Part model, mm, in its own coordinate system. A direction names the side the tool comes from. Round coordinates to 2 decimals unless told otherwise and drop trailing zeros. Write each loop counter-clockwise with the first axis right and the second up, starting at its lowest first coordinate (ties: lowest second). Pieces come first, ordered by that corner, then holes.
```python
from build123d import *

# Parameters (mm, degrees)
F1_DEPTH = 13
F3_DEPTH = 25
F5_DEPTH = 25


with BuildPart() as f1:
    # F0 (on Front) → F1 (new body)
    with BuildSketch(Plane.XZ):
        with BuildLine():
            Line((109.81556, 142.312214), (-107.18444, 142.312214))
            ThreePointArc((-107.18444, 142.312214), (-135.468711, 130.596485), (-147.18444, 102.312214))
            Line((-147.18444, 102.312214), (-147.18444, -27.687786))
            ThreePointArc((-147.18444, -27.687786), (-135.468711, -55.972058), (-107.18444, -67.687786))
            Line((-107.18444, -67.687786), (109.81556, -67.687786))
            ThreePointArc((109.81556, -67.687786), (138.099831, -55.972058), (149.81556, -27.687786))
            Line((149.81556, -27.687786), (149.81556, 102.312214))
            ThreePointArc((149.81556, 102.312214), (138.099831, 130.596485), (109.81556, 142.312214))
        make_face()
    extrude(amount=F1_DEPTH)

    # F2 (on face) → F3 (cut)
    with BuildSketch(Plane.XZ.offset(13)):
        with BuildLine():
            Line((149.81556, -27.687786), (149.81556, -4.202998))
            Line((149.81556, -4.202998), (0, -4.202998))
            Line((0, -4.202998), (0, -30.806687))
            Line((0, -30.806687), (149.693781, -30.806687))
            ThreePointArc((149.693781, -30.806687), (149.785104, -29.248425), (149.81556, -27.687786))
        make_face()
    extrude(amount=-F3_DEPTH, mode=Mode.SUBTRACT)

    # F4 (on face) → F5 (cut)
    with BuildSketch(Plane.XZ.offset(13)):
        with BuildLine():
            Line((36.957689, 109.959573), (149.077729, 109.959573))
            ThreePointArc((149.077729, 109.959573), (147.134331, 116.710454), (144.039855, 123.017229))
            Line((144.039855, 123.017229), (36.957689, 123.017229))
            Line((36.957689, 123.017229), (36.957689, 109.959573))
        make_face()
    extrude(amount=-F5_DEPTH, mode=Mode.SUBTRACT)


solid = f1.part
```
Q1. Mould opens along Z. For faces 3 (the cylindrical face through (-135.156, -6.409, 130.906)), 4 (the flat face through (0, -7, -17)), 5 (the flat face through (149.816, -6, 48)) say: +Z half, -Z half, draft (parallel to the pull), parting line (faces both ways), or undercut.
Values follow:
face 3: +Z half
face 4: undercut
face 5: draft
Q2. Wall check: L1, parallel to Z at x = 64, y = -6.25; L2, parallel to Z at x = 7, y = -2.5; L3, parallel to Z at x = 133, y = -4.5. Give the ranges that are in metal, low to high.
Values follow:
L1: z = -67.69 to -30.81, -4.2 to 109.96, 123.02 to 142.31
L2: z = -67.69 to -30.81, -4.2 to 142.31
L3: z = -60.28 to -30.81, -4.2 to 109.96, 123.02 to 134.91
Q3. Cut at C-C on y = -6. Write the cut outline in (x, z), plus the area to 3 significant figures.
Values follow:
outline: (-147.18, -27.69) arc R40 ccw to (-107.18, -67.69) - (109.82, -67.69) arc R40 ccw to (149.69, -30.81) - (0, -30.81) - (0, -4.2) - (149.82, -4.2) - (149.82, 102.31) arc R40 ccw to (149.08, 109.96) - (36.96, 109.96) - (36.96, 123.02) - (144.04, 123.02) arc R40 ccw to (109.82, 142.31) - (-107.18, 142.31) arc R40 ccw to (-147.18, 102.31) - close
area: 55,600 mm2
Q4. Cut at A-A on x = 100. Write the cut outline in (y, z).
Values follow:
outline: (-13, -67.69) - (0, -67.69) - (0, -30.81) - (-13, -30.81) - close; (-13, -4.2) - (0, -4.2) - (0, 109.96) - (-13, 109.96) - close; (-13, 123.02) - (0, 123.02) - (0, 142.31) - (-13, 142.31) - close
Q5. Which spindle directions (+Z, -Z, +X, -X, +Y, -Y) get a long thin tool onto all of the face, cutting with end or side? Do faces 1 (the flat face through (-147.184, -6, 38)), 2 (the flat face through (91, -7, 123.017)). Say none if no direction does.
Values follow:
face 1: +Z, -Z, -X, +Y, -Y
face 2: +X, +Y, -Y
Q6. Cut at D-D on z = -17. Write the cut outline in (x, y).
Values follow:
outline: (-147.18, -13) - (0, -13) - (0, 0) - (-147.18, 0) - close
Q7. Drop a flat-ended pin along its axis: pin 1 (6.5 mm diameter, centred on y = -9.5, z = 118, fed in from +X). Give the stop position or say it passes through.
Values follow:
pin 1: stops at x = 36.96
Q8. Cut at B-B on x = 10. Write the cut outline in (y, z).
Values follow:
outline: (-13, -67.69) - (0, -67.69) - (0, -30.81) - (-13, -30.81) - close; (-13, -4.2) - (0, -4.2) - (0, 142.31) - (-13, 142.31) - close
